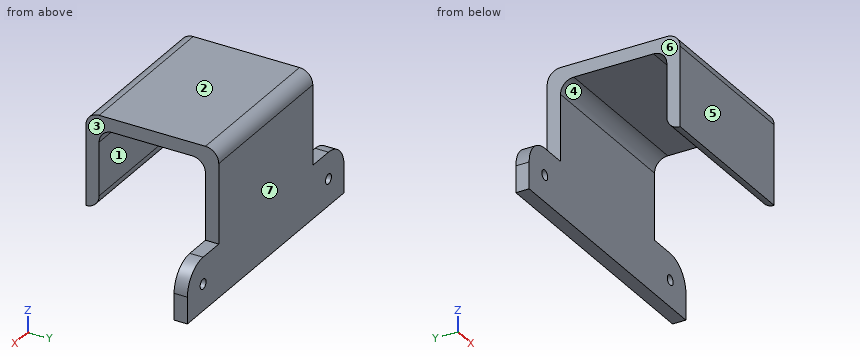
from build123d import *

# Parameters (mm, degrees)
F1_DEPTH = 6.35
F2_R     = 12.7
F4_DEPTH = 38.1
F5_R     = 6.34999


# Not quite as in the source:
# - a fillet or chamfer is up to 0.001 mm smaller than in the source, because OpenCascade refuses the exact size


with BuildPart() as f1:
    # F0 (on Front) → F1 (new body)
    with BuildSketch(Plane.XZ):
        with BuildLine():
            Line((63.5, 0), (63.5, 12.7))
            Line((63.5, 12.7), (-63.5, 12.7))
            Line((-63.5, 12.7), (-63.5, 0))
            Line((-63.5, 0), (-53.18125, 0))
            ThreePointArc((-53.18125, 0), (-50.8, 2.38125), (-48.41875, 0))
            Line((-48.41875, 0), (48.41875, 0))
            ThreePointArc((48.41875, 0), (50.8, 2.38125), (53.18125, 0))
            Line((53.18125, 0), (63.5, 0))
        make_face()
        with BuildLine():
            Line((63.5, -12.7), (63.5, 0))
            Line((63.5, 0), (53.18125, 0))
            ThreePointArc((53.18125, 0), (50.8, -2.38125), (48.41875, 0))
            Line((48.41875, 0), (-48.41875, 0))
            ThreePointArc((-48.41875, 0), (-50.8, -2.38125), (-53.18125, 0))
            Line((-53.18125, 0), (-63.5, 0))
            Line((-63.5, 0), (-63.5, -12.7))
            Line((-63.5, -12.7), (63.5, -12.7))
        make_face()
    extrude(amount=F1_DEPTH)

    # F2
    f2_edges = [f1.edges().sort_by_distance(p)[0] for p in [
        (-63.5, -3.175, 12.7),
        (63.5, -3.175, 12.7),
    ]]
    fillet(f2_edges, radius=F2_R)

    # F3 (on Right) → F4 (join, symmetric)
    with BuildSketch(Plane.YZ):
        Polygon((0, 12.7), (0, 57.15), (-63.5, 57.15), (-63.5, 12.7), (-57.15, 12.7), (-57.15, 50.8), (-6.35, 50.8), (-6.35, 12.7), align=None)
    extrude(amount=F4_DEPTH, both=True)

    # F5 (radius 6.35 in the source; OpenCascade refuses exactly that, so slightly less here)
    f5_edges = [f1.edges().sort_by_distance(p)[0] for p in [
        (0, 0, 57.15),
        (0, -63.5, 57.15),
        (0, -6.35, 50.8),
        (0, -57.15, 50.8),
        (0, -57.15, 12.7),
    ]]
    fillet(f5_edges, radius=F5_R)


solid = f1.part
Build history of the part. All positions in model axes, mm. Face numbers are marked on the shaded views. A direction names the side the tool comes from. Coordinates: 2 decimals unless noted, no trailing zeros. Write each loop counter-clockwise with the first axis right and the second up, starting at its lowest first coordinate (ties: lowest second). Pieces come first, ordered by that corner, then holes.
(1) Mould opens along Y. For the marked faces 4, 5, 6 and 7 say: pulls with the +Y half, pulls with the -Y half, needs draft (parallel to the pull), parting line crosses it, or undercut.
(2) Pin check, flat tips, straight feed: pin 1 Ø22 at (y, z) = (-27.5, 30) entering from +X; pin 2 Ø7 at (x, y) = (43, -3.5) entering from +Z. Stop position of each tip, or through.
(3) Cut at D-D on y = -54. List the corners of the cut face in (x, z).
(4) Cut at B-B on z = 15. List the corners of the cut face in (x, y), and give its area (3 significant figures).
(5) 3-axis set-ups, long thin cutter, end or side, ignore diameter. For the marked faces 1, 2 and 3: which of +Z, -Z, +X, -X, +Y, -Y reach the whole face in a straight line?
(6) Cut at C-C on y = -35.5. List the corners of the cut face in (x, z).
(7) Drill centre lines: line 1 (Y direction, x = 16.5, z = 19); line 2 (Z direction, x = -50.8, y = -2); line 3 (Z direction, x = -18.5, y = -31). Where is each one in solid material? Low to high.
Working result:
1. face 4: undercut
1. face 5: pulls with the -Y half
1. face 6: needs draft
1. face 7: pulls with the +Y half
2. pin 1: passes through
2. pin 2: stops at z = 12.7
3. outline: (-38.1, 49.93) - (38.1, 49.93) - (38.1, 57.15) - (-38.1, 57.15) - close
4. outline: (-38.1, -63.5) - (38.1, -63.5) - (38.1, -58.61) - (-38.1, -58.61) - close; (-38.1, -6.35) - (38.1, -6.35) - (38.1, 0) - (-38.1, 0) - close
4. area: 857 mm2
5. face 1: -Z, +X, -X
5. face 2: +Z, +X, -X, +Y, -Y
5. face 3: +Z, +X, +Y, -Y
6. outline: (-38.1, 50.8) - (38.1, 50.8) - (38.1, 57.15) - (-38.1, 57.15) - close
7. line 1: y = -63.5 to -57.15, -6.35 to 0
7. line 2: z = -12.7 to -2.38, 2.38 to 12.7
7. line 3: z = 50.8 to 57.15
